Input: part model. Units: mm. Frame: model coordinates. A direction names the side the tool comes from. Coordinates: 2 decimals unless noted, no trailing zeros. Order: outer loops, then holes, each group sorted by start corner. A loop starts at its lowest first (then second) coordinate and runs counter-clockwise, first axis right, second up. Notation, with made-up numbers: (40.25, 54.25) -> (92.25, 54.25) arc R28 ccw to (92.25, 92.25) -> close; hole circle Ø5 at (24.5, 45.25). An arc over 180 degrees is marked (long way). Use one line per item in the form item = value. Start each with the question number.
1) Draft query along X for faces 6 (the flat face through (4.5, -7.4, -18.3)), 7 (the flat face through (95.7, -7.6, -9.4)), 8 (the flat face through (0, 0, 0)). Return one class per face: pulls with the +X half, pulls with the -X half, needs draft (parallel to the pull), parting line crosses it, or undercut.
2) Section query B-B on z = -7. Output: boundary loops of the cut face in (x, y), then the cut area to 3 significant figures.
3) Section query A-A on x = 81. Output: boundary loops of the cut face in (y, z).
4) Section query C-C on y = 0.75. Output: boundary loops of the cut face in (x, z), then the cut area to 3 significant figures.
5) Ray query, line 1 along X through (y, z) = (3.75, -3.5); line 2 along X through (y, z) = (-0.75, -57.5); line 3 along Z through (x, y) = (60.5, 4.25). Return the intervals inside material, ascending.
6) Access query for faces 1 (the flat face through (14, 7.6, -53.1)), 2 (the flat face through (-4.5, 7.4, -19.5)), 3 (the flat face through (86.84, -7.39, -10.17)), 4 (the flat face through (80.82, 7.61, -48.95)), 5 (the flat face through (14.257, -7.387, -52.801)). Directions: +Z, -Z, +X, -X, +Y, -Y. A direction counts if a zero-diameter tool reaches every point of the face in a straight line with its end or side. Return the directions, or none.
7) Section query D-D on x = 58. Output: boundary loops of the cut face in (y, z), then the cut area to 3 significant figures.
8) Pin query (flat end, axial travel): pin 1 (5 mm diameter, centred on x = 5.5, y = -3, fed in from +Z); pin 2 (2 mm diameter, centred on y = 5.5, z = -54, fed in from -X); pin 3 (1.5 mm diameter, centred on x = 35.5, y = 3, fed in from +Z). Return the tip coordinate at first contact, or that it passes through.
from build123d import *


with BuildPart() as part:
    # Sweep2: sweep along a path in Sketch3
    with BuildLine(Plane(origin=(0, 0, 0), x_dir=(1, 0, 0), z_dir=(0, 1, 0))) as sweep2_path:
        Line((0, 0), (0, 36.242190507))
        Line((0, 36.242190507), (20.360781184, 73.298812262))
        Line((20.360781184, 73.298812262), (70.448302897, 73.298812262))
        Line((70.448302897, 73.298812262), (97.837038373, 29.582176791))
        Line((97.837038373, 29.582176791), (84.672762234, -11.296364903))
    # Sketch1 → Sweep2 (sweep)
    with BuildSketch(Plane.XY):
        Polygon((8.824071359, -4.70486606), (8.486569209, 5.289436932), (-0.33750215, 9.994302992), (-8.824071359, 4.70486606), (-8.486569209, -5.289436932), (0.33750215, -9.994302992), align=None)
    sweep(path=sweep2_path.line, transition=Transition.RIGHT)


solid = part.part
Answers below:
q1.face_6 = undercut
q1.face_7 = pulls with the +X half
q1.face_8 = needs draft
q2.outline = (-8.82, 4.7) -> (-8.49, -5.29) -> (0.34, -9.99) -> (8.82, -4.7) -> (8.49, 5.29) -> (-0.34, 9.99) -> close; (81.29, -4.7) -> (90.21, -9.99) -> (99.48, -5.29) -> (99.84, 4.7) -> (90.92, 9.99) -> (81.65, 5.29) -> close
q2.area = 533 mm^2
q3.outline = (-9.99, -55.82) -> (-5.29, -72.44) -> (4.7, -73.08) -> (9.99, -57.09) -> (5.29, -40.47) -> (-4.7, -39.84) -> close; (-7.8, 10.11) -> (-4.7, -6.09) -> (5.29, -4.98) -> (7.76, 10.11) -> close
q4.outline = (-8.69, -38.47) -> (15.22, -81.99) -> (75.26, -81.99) -> (107.35, -30.77) -> (92.94, 13.96) -> (76.45, 8.65) -> (88.38, -28.4) -> (65.67, -64.66) -> (25.47, -64.66) -> (8.64, -34.02) -> (8.64, 0) -> (-8.69, 0) -> close
q4.area = 3,870 mm^2
q5.line_1 = -8.79 to 8.54, 80.47 to 98.67
q5.line_2 = 1.82 to 21.6, 70.09 to 90.54
q5.line_3 = -82.11 to -64.78
q6.face_1 = +Z, +Y
q6.face_2 = +Z, -Z, -X, +Y
q6.face_3 = -Y
q6.face_4 = +Y
q6.face_5 = +Z, -Y
q7.outline = (-9.99, -72.96) -> (-5.29, -81.79) -> (4.7, -82.12) -> (9.99, -73.64) -> (5.29, -64.81) -> (-4.7, -64.47) -> close
q7.area = 260 mm^2
q8.pin_1 = 0
q8.pin_2 = -0.64
q8.pin_3 = -64.71
